Autodesk Inventor part; units mm, degrees
ref_plane "YZ Plane" through (0, 0, 0) normal (1, 0, 0) x (0, 1, 0)
ref_plane "XZ Plane" through (0, 0, 0) normal (0, 1, 0) x (-1, 0, 0)
ref_plane "XY Plane" through (0, 0, 0) normal (0, 0, 1) x (1, 0, 0)
sketch "スケッチ1" plane through (0, 0, 0) normal (0, 0, 1) x (1, 0, 0)
  line L0 (0, 0) -> (300, 0)
  line L1 (300, 0) -> (300, 175)
  line L2 (300, 175) -> (0, 175)
  line L3 (0, 175) -> (0, 0)
  dimension "d0" = 175
  dimension "d1" = 300
extrude "押し出し1" add sketch "スケッチ1" along normal blind 3
sketch "スケッチ2" plane through (0, 0, 3) normal (0, 0, 1) x (1, 0, 0)
  line L0 (-6.3861, 0) -> (323.6139, 0)
  circle A0 centre (75, 60) radius 46
  circle A1 centre (225, 60) radius 46
  line L1 (75, 60) -> (75, 156.1238)
  line L2 (225, 60) -> (225, 147.3766)
  line L3 (75, 60) -> (50.2691, 119.7057)
  line L4 (225, 60) -> (203.3576, 112.2494)
  circle A2 centre (57.3966, 102.4985) radius 1.6
  circle A3 centre (207.3966, 102.4985) radius 1.6
  circle A4 centre (32.5015, 77.6034) radius 1.6
  circle A5 centre (32.5015, 42.3966) radius 1.6
  circle A6 centre (57.3966, 17.5015) radius 1.6
  circle A7 centre (92.6034, 17.5015) radius 1.6
  circle A8 centre (117.4985, 42.3966) radius 1.6
  circle A9 centre (117.4985, 77.6034) radius 1.6
  circle A10 centre (92.6034, 102.4985) radius 1.6
  circle A11 centre (182.5015, 77.6034) radius 1.6
  circle A12 centre (182.5015, 42.3966) radius 1.6
  circle A13 centre (207.3966, 17.5015) radius 1.6
  circle A14 centre (242.6034, 17.5015) radius 1.6
  circle A15 centre (267.4985, 42.3966) radius 1.6
  circle A16 centre (267.4985, 77.6034) radius 1.6
  circle A17 centre (242.6034, 102.4985) radius 1.6
  circle A18 centre (75, 60) radius 30
  circle A19 centre (225, 60) radius 30
  line L5 (323.6139, 175) -> (-6.3861, 175)
  line L6 (-6.3861, 145) -> (19.1813, 0)
  line L7 (323.6139, 145) -> (298.0465, 0)
  line L8 (0, 175) -> (0, 0)
  line L9 (300, 175) -> (300, 0)
  line L10 (300, 175) -> (0, 175)
  line L11 (0, 175) -> (0, 0)
  dimension "d10" = 92
  dimension "d11" = 92
  dimension "d8" = 60
  dimension "d9" = 60
  dimension "d12" = 22.5
  dimension "d13" = 22.5
  dimension "d14" = 3.2
  dimension "d15" = 3.2
  dimension "d16" = 360
  dimension "d17" = 360
  dimension "d18" = 60
  dimension "d19" = 60
  dimension "d20" = 175
  dimension "d21" = 30
  dimension "d22" = 30
  dimension "d23" = 80
  dimension "d24" = 80
  dimension "d25" = 300
  dimension "d26" = 0
  dimension "d27" = 0
  dimension "d28" = 150
  dimension "d29" = 75
extrude "押し出し2" cut sketch "スケッチ2" against normal blind 5 contours A9 A0 | A0 A9 | A8 A0 | A0 A8 | A7 A0 | A0 A7 | A6 A0 | A0 A6 | A18 L3 L1 | L1 L3 A18 | A5 A0 | A0 A5 | A4 A0 | A0 A4 | A16 A1 | A1 A16 | A15 A1 | A1 A15 | A14 A1 | A1 A14 | A13 A1 | A1 A13 | A19 L4 L2 | L2 L4 A19 | A12 A1 | A1 A12 | A11 A1 | A1 A11
sketch "スケッチ3" plane through (0, 0, 3) normal (0, 0, 1) x (1, 0, 0)
  circle A0 centre (75, 60) radius 30
  line L0 (75, 60) -> (100, 60)
  line L1 (100, 60) -> (100, 110)
  line L2 (100, 110) -> (75, 110)
  line L3 (75, 110) -> (75, 60)
  line L4 (75, 110) -> (50, 110)
  line L5 (50, 110) -> (50, 60)
  line L6 (50, 60) -> (75, 60)
  line L7 (75, 60) -> (75, 110)
  line L8 (50, 110) -> (42.3811, 36.1629)
  line L9 (100, 110) -> (107.6189, 36.1629)
  line L10 (300, 175) -> (0, 175)
  line L11 (150, 175) -> (150, 0)
  line L12 (0, 0) -> (300, 0)
  line L13 (200, 110) -> (225, 110)
  line L14 (225, 110) -> (250, 110)
  line L15 (250, 110) -> (257.6189, 36.1629)
  line L16 (200, 110) -> (192.3811, 36.1629)
  circle A1 centre (225, 60) radius 30
  circle A2 centre (225, 60) radius 30
  point P0 (45.1584, 63.0792)
  point P1 (104.8416, 63.0792)
  point P2 (195.1584, 63.0792)
  point P3 (254.8416, 63.0792)
  dimension "d32" = 25
  dimension "d33" = 50
  dimension "d34" = 25
extrude "押し出し3" cut sketch "スケッチ3" against normal blind 5 contours A0 L1 L9 | L8 L5 A0 | A0 L3 L2 L1 | L5 L4 L3 A0 | L13 L14 L15 A1 L16
sketch "スケッチ4" plane through (0, 0, 3) normal (0, 0, 1) x (1, 0, 0)
  line L0 (0, 175) -> (0, 0)
  line L1 (300, 0) -> (300, 175)
  line L2 (0, 175) -> (300, 175)
  line L3 (300, 175) -> (300, 110)
  line L4 (300, 110) -> (0, 110)
  line L5 (0, 110) -> (0, 175)
  line L6 (0, 147) -> (300, 147)
  line L7 (300, 147) -> (300, 117)
  line L8 (300, 117) -> (0, 117)
  line L9 (0, 117) -> (0, 147)
  line L10 (40, 147) -> (110, 147)
  line L11 (110, 147) -> (110, 117)
  line L12 (110, 117) -> (40, 117)
  line L13 (40, 117) -> (40, 147)
  line L14 (150, 117) -> (150, 0)
  line L15 (190, 147) -> (190, 117)
  line L16 (260, 117) -> (260, 147)
  point P0 (110, 147)
  dimension "d38" = 65
  dimension "d39" = 30
  dimension "d40" = 7
  dimension "d41" = 70
  dimension "d192" = 40
extrude "押し出し4" cut sketch "スケッチ4" against normal blind 5 contours L6 L11 L8 L13 | L16 L8 L15 L6
fillet "フィレット2" radius 5 12 edges at (110, 147, 1.5) (260, 147, 1.5) (260, 117, 1.5) (190, 147, 1.5) (190, 117, 1.5) (40, 117, 1.5) (40, 147, 1.5) (110, 117, 1.5) (100, 110, 1.5) (250, 110, 1.5) (200, 110, 1.5) (50, 110, 1.5)
sketch "スケッチ5" plane through (0, 0, 3) normal (0, 0, 1) x (1, 0, 0)
  line L0 (300, 175) -> (0, 175)
  line L1 (300, 0) -> (300, 175)
  line L2 (0, 175) -> (300, 175)
  line L3 (300, 175) -> (300, 170)
  line L4 (300, 170) -> (0, 170)
  line L5 (0, 170) -> (0, 175)
  line L6 (20, 175) -> (20, 170)
  line L7 (40, 175) -> (40, 170)
  line L8 (60, 175) -> (60, 170)
  line L9 (80, 175) -> (80, 170)
  line L10 (100, 175) -> (100, 170)
  line L11 (120, 175) -> (120, 170)
  line L12 (140, 175) -> (140, 170)
  line L13 (160, 175) -> (160, 170)
  line L14 (180, 175) -> (180, 170)
  line L15 (200, 175) -> (200, 170)
  line L16 (220, 175) -> (220, 170)
  line L17 (240, 175) -> (240, 170)
  line L18 (260, 175) -> (260, 170)
  line L19 (280, 175) -> (280, 170)
  line L20 (300, 175) -> (300, 170)
  point P0 (0, 0)
  point P1 (0, 172.5)
  dimension "d46" = 5
  dimension "d47" = 20
  dimension "d50" = 20
extrude "押し出し5" cut sketch "スケッチ5" against normal blind 5
fillet "フィレット6" radius 10 2 edges at (0, 0, 1.5) (300, 0, 1.5)
fillet "フィレット7" radius 2 2 edges at (300, 170, 1.5) (0, 170, 1.5)
sketch "スケッチ12" plane through (0, 0, 3) normal (0, 0, 1) x (1, 0, 0)
  line L0 (298, 170) -> (2, 170)
  line L1 (150, 170) -> (150, 0)
  line L2 (10, 0) -> (290, 0)
  line L3 (300, 10) -> (300, 168)
  line L4 (0, 168) -> (0, 10)
  point P0 (0, 0)
  point P1 (150, 40)
  point P2 (150, 80)
  point P3 (150, 120)
  dimension "d194" = 300
  dimension "d195" = 150
  dimension "d196" = 40
  dimension "d197" = 40
  dimension "d198" = 40
hole "穴3" at (150, 40, 3) at (150, 80, 3) at (150, 120, 3) direction (0, 0, -1) diameter 5.2 end through all
sketch "スケッチ14" plane through (0, 0, 0) normal (0, 0, -1) x (-1, 0, 0)
  line L0 (-300, 10) -> (-300, 168)
  line L1 (-300, 160) -> (0, 160)
  line L2 (0, 168) -> (0, 10)
  line L3 (-2, 170) -> (-298, 170)
  point P0 (0, 0)
  point P1 (-150, 160)
  point P2 (-200, 160)
  point P3 (-250, 160)
  point P4 (-100, 160)
  point P5 (-50, 160)
  dimension "d220" = 10
  dimension "d221" = 150
  dimension "d222" = 50
  dimension "d223" = 50
  dimension "d224" = 50
  dimension "d225" = 50
hole "穴4" at (150, 160, 0) at (200, 160, 0) at (250, 160, 0) at (100, 160, 0) at (50, 160, 0) direction (0, 0, 1) diameter 5.2 end through all
equation "\"d11\" = d10"
equation "\"d8\" = d9"
equation "\"d15\" = d14"
equation "\"d24\" = d23"
equation "\"d34\" = d32"
properties part number "RP_Waist-Under-ver2" material "アルミニウム 6061"
For this review, take the finished solid that the model builds, in its own axes (mm). Round coordinates to 2 decimals unless told otherwise and drop trailing zeros. Write each loop counter-clockwise with the first axis right and the second up, starting at its lowest first coordinate (ties: lowest second). Pieces come first, ordered by that corner, then holes. Notation, with made-up numbers: (10, 54.5) - (54, 54.5) arc R18 ccw to (54, 62.5) - close; hole circle Ø2 at (32, 82.25). An arc over 180 degrees is marked (long way). Use a Markdown table: item, result.
Q1. Clearance check with a flat-ended pin moving along its axis: pin 1 (1.9 mm diameter, centred on x = 182.5, y = 42.4, fed in from -Z). State where the tip first meets the part, or that it passes through.
Derived:
| item | result |
|---|---|
| pin 1 | passes through |
Q2. Wall thickness on line 1 along X through (y, z) = (160, 1.75); line 2 along Y through (x, z) = (77, 1.1); line 3 along X through (y, z) = (63, 1.6): over which ranges is each line inside the solid? List them lowest first.
Derived:
| item | result |
|---|---|
| line 1 | x = 0 to 47.4, 52.6 to 97.4, 102.6 to 147.4, 152.6 to 197.4, 202.6 to 247.4, 252.6 to 300 |
| line 2 | y = 0 to 30.07, 110 to 117, 147 to 170 |
| line 3 | x = 0 to 45.15, 104.85 to 195.15, 254.85 to 300 |
Q3. We need section A-A (x = 75). Give the boundary of the cut face in (y, z), plus the area to 3 significant figures.
Derived:
| item | result |
|---|---|
| outline | (0, 0) - (30, 0) - (30, 3) - (0, 3) - close; (110, 0) - (117, 0) - (117, 3) - (110, 3) - close; (147, 0) - (170, 0) - (170, 3) - (147, 3) - close |
| area | 180 mm2 |
Q4. We need section B-B (y = 60). Give the boundary of the cut face in (x, z).
Derived:
| item | result |
|---|---|
| outline | (0, 0) - (45, 0) - (45, 3) - (0, 3) - close; (105, 0) - (195, 0) - (195, 3) - (105, 3) - close; (255, 0) - (300, 0) - (300, 3) - (255, 3) - close |
Q5. We need section C-C (z = 1.5). State how many separate pieces and enclosed holes the cut face has, plus the area to 3 significant figures.
Derived:
| item | result |
|---|---|
| separate pieces | 1 |
| enclosed holes | 24 |
| area | 38,200 mm2 |
Q6. The part is to be moulded in two halves that separate along X. For faces 1 (the flat face through (148, 86, 0)), 2 (the cylindrical face through (2.85, 3.01, 1.52)), 3 (the cylindrical face through (296.99, 2.85, 1.52)), 4 (the cylindrical face through (151, 117.6, 1.5)), say which applies: pulls with the +X half, pulls with the -X half, needs draft (parallel to the pull), parting line crosses it, or undercut.
Derived:
| item | result |
|---|---|
| face 1 | needs draft |
| face 2 | pulls with the -X half |
| face 3 | pulls with the +X half |
| face 4 | undercut |
